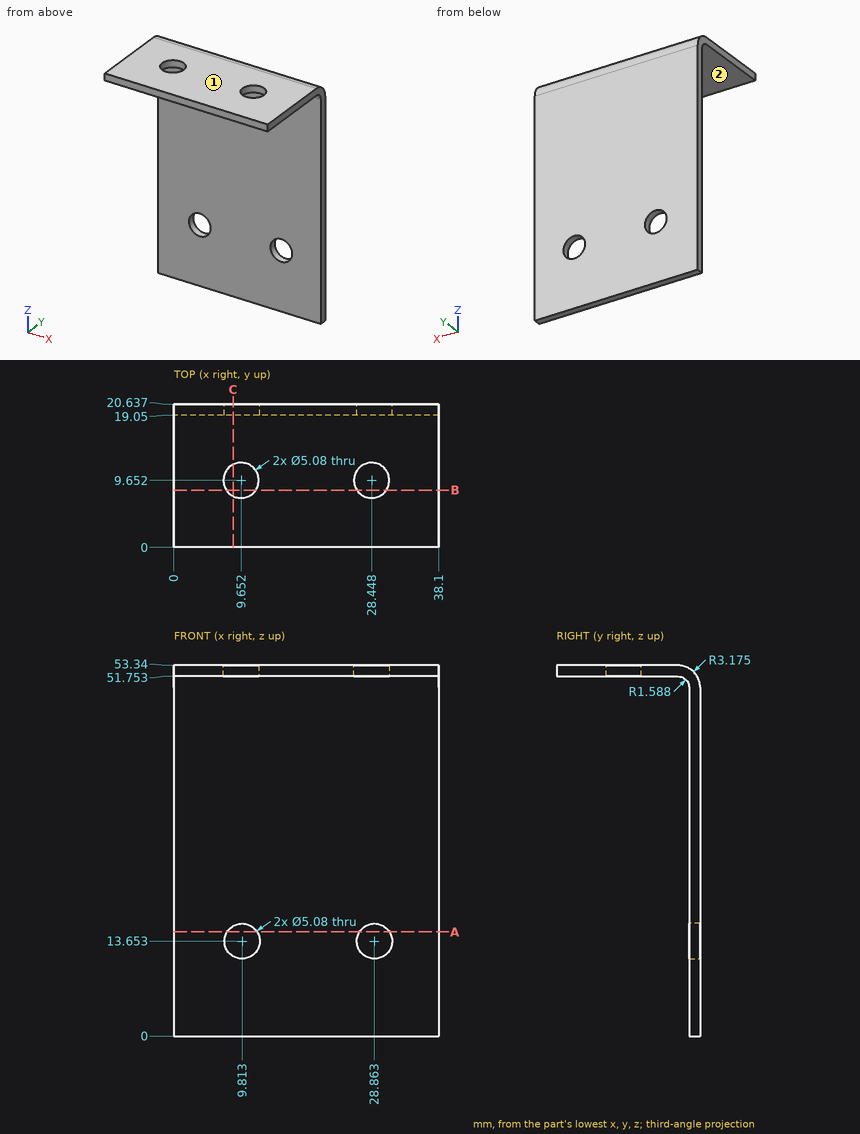
Design review of the part shown in the three views and the two pictorial views. Dimensions are in mm from the part's minimum x, y and z. A direction names the side the tool comes from. Coordinates: 2 decimals unless noted, no trailing zeros. Write each loop counter-clockwise with the first axis right and the second up, starting at its lowest first coordinate (ties: lowest second). Pieces come first, ordered by that corner, then holes. Notation, with made-up numbers: (10.25, -39) - (27.25, -39) arc R18 cw to (27.25, -11) - close; hole circle Ø9 at (61.5, 29.5). An arc over 180 degrees is marked (long way). Write item = value, one per line.
(1) For P1, Ø5, axis at x = 24, y = 4.5, coming from the -Z side, flat-tipped, find the tip position at first contact; note if it passes through.
Result sheet:
P1 = 51.75
(2) Machinability: for the marked faces 1 and 2, which of the approach directions +Z, -Z, +X, -X, +Y, -Y give a long, thin tool a straight path to every point of the face, cutting with its end or side? Answer none if there is none.
Result sheet:
face_1 = +Z, +X, -X, +Y, -Y
face_2 = -Z, +X, -X, -Y
(3) Consider section C-C, the plane x = 8.5. State how many separate pieces and enclosed holes the cut face has.
Result sheet:
separate_pieces = 3
enclosed_holes = 0
(4) For line 1 (Y direction, x = 15, z = 20.5); line 2 (Z direction, x = 31, y = 5); line 3 (Z direction, x = 20.5, y = 18.75) (1 decimal), list the stretches that pass through material, from the lowest coordinate up. Write a range as [from, to].
Result sheet:
line_1 = [19.05, 20.64]
line_2 = [51.75, 53.34]
line_3 = [51.1, 53.1]
(5) Consider section B-B, the plane y = 8.25. Give the boundary of the cut face in (x, z).
Result sheet:
outline = (0, 51.75) - (7.53, 51.75) - (7.53, 53.34) - (0, 53.34) - close; (11.77, 51.75) - (26.33, 51.75) - (26.33, 53.34) - (11.77, 53.34) - close; (30.57, 51.75) - (38.1, 51.75) - (38.1, 53.34) - (30.57, 53.34) - close
(6) Consider section A-A, the plane z = 15. Give the boundary of the cut face in (x, y).
Result sheet:
outline = (0, 19.05) - (7.66, 19.05) - (7.66, 20.64) - (0, 20.64) - close; (11.97, 19.05) - (26.71, 19.05) - (26.71, 20.64) - (11.97, 20.64) - close; (31.02, 19.05) - (38.1, 19.05) - (38.1, 20.64) - (31.02, 20.64) - close
